from build123d import *

# Parameters (mm, degrees)
SKETCH_R   = 3
SKETCH_R_2 = 1.5
PAD_DEPTH  = 3


with BuildPart() as part:
    # Sketch → Pad (new body)
    with BuildSketch(Plane.XY):
        Polygon((87, 0), (87, 91.15), (17, 91.15), (17, 30.85), (0, 30.85), (0, 11.5), (11.5, 11.5), (11.5, 0), align=None)
        with Locations((27, 74.15)):
            Circle(SKETCH_R, mode=Mode.SUBTRACT)
        with Locations((58, 74.15)):
            Circle(SKETCH_R, mode=Mode.SUBTRACT)
        with Locations((58, 43.85)):
            Circle(SKETCH_R, mode=Mode.SUBTRACT)
        with Locations((27, 43.85)):
            Circle(SKETCH_R, mode=Mode.SUBTRACT)
        with Locations((21.7, 5)):
            Circle(SKETCH_R_2, mode=Mode.SUBTRACT)
        with Locations((29.7, 5)):
            Circle(SKETCH_R_2, mode=Mode.SUBTRACT)
        with Locations((70.3, 8.7)):
            Circle(SKETCH_R_2, mode=Mode.SUBTRACT)
        with Locations((62.3, 8.7)):
            Circle(SKETCH_R_2, mode=Mode.SUBTRACT)
        with Locations((22.7, 85.45)):
            Circle(SKETCH_R_2, mode=Mode.SUBTRACT)
        with Locations((67, 85.45)):
            Circle(SKETCH_R_2, mode=Mode.SUBTRACT)
        Polygon((68, 59), (68, 66.5), (53, 66.5), (53, 51.5), (68, 51.5), align=None, mode=Mode.SUBTRACT)
    pad = extrude(amount=PAD_DEPTH)

    # Mirrored: Pad across face of Pad
    add(pad.mirror(Plane(origin=(87, 45.575, 1.5), x_dir=(0, 1, 0), z_dir=(1, 0, 0))))


solid = part.part
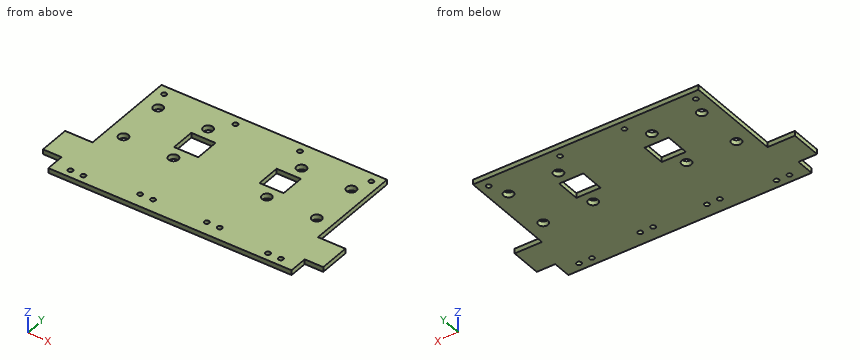
Work out the finished part from the listing and answer in its coordinate system (mm). Coordinates: 2 decimals unless noted, no trailing zeros. Loops run counter-clockwise (first coordinate to the right, second up) from the corner with the lowest first, then second, coordinate; pieces in that order, holes last. Notation, with made-up numbers: M 65,41.5 L 101,41.5 A15 cw 101,59.5 Z; hole C 35.5,-3.75 d3. An arc over 180 degrees is marked long. Answer in a Markdown table with one row per item. Add a question column.
1. Find section B-B, the plane z = 1.1. State how many separate pieces and enclosed holes the cut face has, then the cut area to 3 significant figures.
2. Flat-ended cylindrical pins translate along their axes: P1, Ø9.5, axis at x = 27, y = 43.85, coming from the +Z side; P2, Ø1.5, axis at y = 10, z = 1.5, coming from the -X side; P3, Ø1.5, axis at y = 3, z = 1, coming from the +X side; P4, Ø1.5, axis at y = 56.5, z = 1.5, coming from the -X side. Find the tip coordinate at first contact, or state that the pin passes through.
3. Consider L1, parallel to X at y = 61.5, z = 1.3; L2, parallel to X at y = 43.5, z = 2.6; L3, parallel to Y at x = 67, z = 1.95. Determine where each line is inside the solid, lowest interval first.
4. Find section C-C, the plane y = 79. Write down the section's boundary in (x, z), then the cut area to 3 significant figures.
5. Find section A-A, the plane y = 56. Write down the section's boundary in (x, z).
Reported:
| question | item | result |
|---|---|---|
| 1 | separate pieces | 1 |
| 1 | enclosed holes | 22 |
| 1 | area | 12,800 mm^2 |
| 2 | P1 | stops at z = 3 |
| 2 | P2 | stops at x = 11.5 |
| 2 | P3 | stops at x = 162.5 |
| 2 | P4 | stops at x = 17 |
| 3 | L1 | x = 17 to 53, 68 to 106, 121 to 157 |
| 3 | L2 | x = 17 to 24.02, 29.98 to 55.02, 60.98 to 113.02, 118.98 to 144.02, 149.98 to 157 |
| 3 | L3 | y = 0 to 51.5, 66.5 to 83.95, 86.95 to 91.15 |
| 4 | outline | M 17,0 L 157,0 L 157,3 L 17,3 Z |
| 4 | area | 420 mm^2 |
| 5 | outline | M 17,0 L 53,0 L 53,3 L 17,3 Z; M 68,0 L 106,0 L 106,3 L 68,3 Z; M 121,0 L 157,0 L 157,3 L 121,3 Z |
